Work out the finished part from the listing and answer in its coordinate system (mm). A direction names the side the tool comes from. Give positions to 0.01 mm unless a question says otherwise; leave off trailing zeros. Write each loop counter-clockwise with the first axis right and the second up, starting at its lowest first coordinate (ties: lowest second). Pieces come first, ordered by that corner, then holes. Notation, with made-up numbers: (82.5, 27.5) - (123.5, 27.5) arc R6 ccw to (123.5, 38.5) - close; hole circle Ø10 at (-33.5, -1.75). An arc over 180 degrees is marked (long way). Write each question's results on one line, items separated by ' | '. Start each with the question number.
from build123d import *

# Parameters (mm, degrees)
SKETCH1_W               = 48
SKETCH1_H               = 10
BOSS_EXTRUDE5_DEPTH     = 2
BOSS_EXTRUDE6_START     = 5
BOSS_EXTRUDE6_DEPTH     = 2
SKETCH3_R               = 8.25
CUT_EXTRUDE1_DEPTH      = 2
CUT_EXTRUDE2_DEPTH      = 40.051403925
CUT_EXTRUDE2_DEPTH_BACK = 40.051403925
CUT_EXTRUDE3_DEPTH      = 40.051403925
CUT_EXTRUDE3_DEPTH_BACK = 10
SKETCH6_R               = 1.2
SKETCH6_R_2             = 1.211894006


with BuildPart() as part:
    # Sketch1 → Boss-Extrude5 (new body)
    with BuildSketch(Plane.XY):
        Rectangle(SKETCH1_W, SKETCH1_H)
    extrude(amount=-BOSS_EXTRUDE5_DEPTH)

    # Sketch2 → Boss-Extrude6 (add)
    with BuildSketch(Plane(origin=(0, 0, 0), x_dir=(1, 0, 0), z_dir=(0, 1, 0)).offset(BOSS_EXTRUDE6_START)):
        with BuildLine():
            ThreePointArc((-1.241034606, 23.712139016), (-12, 30.397568135), (-22.758965394, 23.712139016))
            Line((-22.758965394, 23.712139016), (-1.241034606, 23.712139016))
        make_face()
        with BuildLine():
            Line((-1.241034606, 23.712139016), (-22.758965394, 23.712139016))
            ThreePointArc((-22.758965394, 23.712139016), (-23.685623319, 21.126342152), (-24, 18.397568135))
            ThreePointArc((-24, 18.397568135), (-12, 6.397568135), (0, 18.397568135))
            ThreePointArc((0, 18.397568135), (-0.314376681, 21.126342152), (-1.241034606, 23.712139016))
        make_face()
        with BuildLine():
            ThreePointArc((22.758965394, 23.712139016), (12, 30.397568135), (1.241034606, 23.712139016))
            Line((1.241034606, 23.712139016), (22.758965394, 23.712139016))
        make_face()
        with BuildLine():
            Line((22.758965394, 23.712139016), (1.241034606, 23.712139016))
            ThreePointArc((1.241034606, 23.712139016), (0.314376681, 21.126342152), (0, 18.397568135))
            ThreePointArc((0, 18.397568135), (12, 6.397568135), (24, 18.397568135))
            ThreePointArc((24, 18.397568135), (23.685623319, 21.126342152), (22.758965394, 23.712139016))
        make_face()
        with BuildLine():
            ThreePointArc((0, 18.397568135), (-12, 6.397568135), (-24, 18.397568135))
            Line((-24, 18.397568135), (-24, 2))
            Line((-24, 2), (24, 2))
            Line((24, 2), (24, 18.397568135))
            ThreePointArc((24, 18.397568135), (12, 6.397568135), (0, 18.397568135))
        make_face()
    extrude(amount=-BOSS_EXTRUDE6_DEPTH)

    # Sketch3 → Cut-Extrude1 (cut)
    with BuildSketch(Plane(origin=(0, 5, 0), x_dir=(1, 0, 0), z_dir=(0, 1, 0))):
        with Locations(Location((-13.286531406, 15.996474508, 0), (0, 0, 270))):
            Circle(SKETCH3_R)
        with Locations(Location((13.213468594, 15.996474508, 0), (0, 0, 270))):
            Circle(SKETCH3_R)
    extrude(amount=-CUT_EXTRUDE1_DEPTH, mode=Mode.SUBTRACT)

    # Sketch5 → Cut-Extrude2 (cut, two sides: drawn at the far end of the back side and taken through both)
    with BuildSketch(Plane(origin=(0, 0, 0), x_dir=(1, 0, 0), z_dir=(0, 1, 0)).offset(-CUT_EXTRUDE2_DEPTH_BACK)):
        with BuildLine():
            Line((-3.373580641, 7.393929887), (3.026393541, 7.406054321))
            ThreePointArc((3.026393541, 7.406054321), (5.230557377, 5.210226053), (3.034729108, 3.006062217))
            Line((3.034729108, 3.006062217), (-3.365245074, 2.993937783))
            ThreePointArc((-3.365245074, 2.993937783), (-5.56940891, 5.189766052), (-3.373580641, 7.393929887))
        make_face()
    extrude(amount=CUT_EXTRUDE2_DEPTH + CUT_EXTRUDE2_DEPTH_BACK, mode=Mode.SUBTRACT)

    # Sketch6 → Cut-Extrude3 (cut, two sides: drawn at the far end of the back side and taken through both)
    with BuildSketch(Plane.XY.offset(-CUT_EXTRUDE3_DEPTH_BACK)):
        with Locations(Location((-19.864598195, -1.616601086, 0), (0, 0, 180))):
            Circle(SKETCH6_R)
        with Locations(Location((19.86, -1.616601086, 0), (0, 0, 180))):
            Circle(SKETCH6_R_2)
    extrude(amount=CUT_EXTRUDE3_DEPTH + CUT_EXTRUDE3_DEPTH_BACK, mode=Mode.SUBTRACT)


solid = part.part
Q1. A cutting plane is placed at C-C, the plane z = -21. Write down the section's boundary in (x, y), and give its area (3 significant figures).
Q2. The mould has two halves that part along Z. Classify faces 1 (the flat face through (24, 3.4, -7.1)), 2 (the flat face through (0, 0, 0)), 3 (the cylindrical face through (-5.57, 3.99, -5.14)): pulls with the +Z half, pulls with the -Z half, needs draft (parallel to the pull), parting line crosses it, or undercut.
Q3. A cutting plane is placed at A-A, the plane x = 19.86. Write down the section's boundary in (y, z), and give its area (3 significant figures).
Q4. Consider L1, parallel to Y at x = -3, z = -10; L2, parallel to X at y = 3.5, z = -23.5; L3, parallel to X at y = -2.5, z = -1.5. Determine where each line is inside the solid, lowest interval first.
Q5. A tool of negligible diameter and unlimited length cuts with its end or side. For faces 4 (the flat face through (0, 3, -16)), 5 (the cylindrical face through (5.23, 3.99, -5.26)), 6 (the cylindrical face through (-20.973, -1.157, -1.014)), from which of +Z, -Z, +X, -X, +Y, -Y can it reach the whole face along a straight path? Write none if from no direction.
Q6. A cutting plane is placed at D-D, the plane x = -17.5. Write down the section's boundary in (y, z).
Q7. A cutting plane is placed at B-B, the plane y = -1. Write down the section's boundary in (x, z), and give its area (3 significant figures).
Q8. Given pin 1 (1.5 mm diameter, centred on y = 2.5, z = -7.5, fed in from +X); pin 2 (10 mm diameter, centred on x = 15, z = -9.5, fed in from -Y); pin 3 (4 mm diameter, centred on x = 17.5, y = -2.5, fed in from -Z); pin 4 (3 mm diameter, centred on y = 3, z = -25, fed in from +X), each flat-ended and moving along its own axis, determine where each tip first touches the part or whether it passes through.
Result:
1) outline: (-23.71, 3) - (-19.85, 3) - (-19.85, 5) - (-23.71, 5) - close; (-6.73, 3) - (-0.29, 3) - (-0.29, 5) - (-6.73, 5) - close; (0.29, 3) - (6.65, 3) - (6.65, 5) - (0.29, 5) - close; (19.77, 3) - (23.71, 3) - (23.71, 5) - (19.77, 5) - close | area: 41.2 mm2
2) face 1: needs draft | face 2: pulls with the +Z half | face 3: undercut
3) outline: (-5, -2) - (-2.83, -2) - (-2.83, 0) - (-5, 0) - close; (-0.4, -2) - (3, -2) - (3, -11.11) - (5, -11.11) - (5, 0) - (-0.4, 0) - close; (3, -27.47) - (5, -27.47) - (5, -20.88) - (3, -20.88) - close | area: 46.5 mm2
4) L1: y = 3 to 5 | L2: x = -22.86 to -16.72, -9.86 to -1.14, 1.14 to 9.78, 16.64 to 22.86 | L3: x = -24 to -20.68, -19.05 to 19.03, 20.69 to 24
5) face 4: -Z, +X, -X, -Y | face 5: +Y, -Y | face 6: +Z, -Z
6) outline: (-5, -2) - (3, -2) - (3, -8.9) - (5, -8.9) - (5, 0) - (-5, 0) - close; (3, -29.06) - (5, -29.06) - (5, -23.09) - (3, -23.09) - close
7) outline: (-24, -2) - (-20.89, -2) - (-20.89, 0) - (-24, 0) - close; (-18.84, -2) - (18.82, -2) - (18.82, 0) - (-18.84, 0) - close; (20.9, -2) - (24, -2) - (24, 0) - (20.9, 0) - close | area: 87.7 mm2
8) pin 1: stops at x = 24 | pin 2: stops at y = 3 | pin 3: stops at z = -2 | pin 4: stops at x = 22.86
